Autodesk Inventor part; units mm, degrees
ref_plane "YZ Plane" through (0, 0, 0) normal (1, 0, 0) x (0, 1, 0)
ref_plane "XZ Plane" through (0, 0, 0) normal (0, 1, 0) x (-1, 0, 0)
ref_plane "XY Plane" through (0, 0, 0) normal (0, 0, 1) x (1, 0, 0)
sketch "Sketch1" plane through (0, 0, 0) normal (0, 0, 1) x (1, 0, 0)
  line L0 (33.401, 0) -> (-33.401, 0) construction
  arc A0 (33.401, 7.9375) -> (35.033, -7.7679) centre (33.401, 0) ccw construction
  arc A1 (-35.033, -7.7679) -> (-33.401, 7.9375) centre (-33.401, 0) ccw construction
  line L1 (33.401, 7.9375) -> (-33.401, 7.9375)
  line L2 (35.033, -7.7679) -> (19.1135, -11.1125)
  line L3 (19.1135, -11.1125) -> (19.1135, -30.1625)
  line L4 (19.1135, -30.1625) -> (44.5135, -36.9684)
  line L5 (44.5135, -36.9684) -> (44.5135, -81.4184)
  line L6 (44.5135, -81.4184) -> (-19.1135, -42.8625)
  line L7 (-19.1135, -42.8625) -> (-19.1135, -11.1125)
  line L8 (-19.1135, -11.1125) -> (-43.434, -6.0029)
  arc A2 (35.033, -7.7679) -> (33.401, 7.9375) centre (33.401, 0) ccw
  arc A3 (-33.401, 7.9375) -> (-35.033, -7.7679) centre (-33.401, 0) ccw
  line L9 (0, 26.6914) -> (0, -99.4367) construction
  line L10 (-33.401, 7.9375) -> (-43.434, 7.9375)
  line L11 (-43.434, 7.9375) -> (-43.434, -6.0029)
  point P0 (0, 0)
  point P1 (0, 0)
  point P2 (19.1135, -20.6375)
  dimension "d24" = 50.927
  dimension "d25" = 7.9375
  dimension "d26" = 19.05
  dimension "d27" = 19.05
  dimension "d28" = 105
  dimension "d30" = 6.35
  dimension "d31" = 44.45
  dimension "d72" = 28.575
  dimension "d110" = 31.75
  dimension "d127" = 10.033
extrude "Extrusion2" add sketch "Sketch1" along normal mid plane 9.525
sketch "Sketch2" plane through (0, 0, 4.7625) normal (0, 0, 1) x (1, 0, 0)
  arc A0 (35.033, -7.7679) -> (33.401, 7.9375) centre (33.401, 0) ccw construction
  line L0 (33.401, 0) -> (-33.401, 0) construction
  point P0 (0, 0)
  point P1 (0, 0)
hole "Hole1" at (33.401, 0, 4.7625) at (-33.401, 0, 4.7625) direction (0, 0, -1) diameter 3.9624 end through all
sketch "Sketch3" plane through (0, 0, -4.7625) normal (0, 0, -1) x (-1, 0, 0)
  line L0 (-62.103, 0) -> (61.0235, 0) construction
  line L1 (0, -99.2896) -> (0, 25.8087) construction
  line L2 (11.1125, -1.5875) -> (-11.1125, -1.5875) construction
  line L3 (0, -26.9875) -> (0, -1.5875) construction
  point P0 (0, 0)
  dimension "d43" = 22.225
  dimension "d44" = 25.4
  dimension "d45" = 1.5875
hole "Hole2" at (0, -26.9875, -4.7625) at (11.1125, -1.5875, -4.7625) at (-11.1125, -1.5875, -4.7625) direction (0, 0, 1) diameter 3.9624 end through all
sketch "Sketch4" plane through (0, 0, 4.7625) normal (0, 0, 1) x (1, 0, 0)
  line L0 (0, 0) -> (0, -12.7) construction
  circle A0 centre (0, -12.7) radius 9.525
  line L1 (25.4635, -56.9863) -> (25.4635, -41.6407)
  line L2 (23.9574, -39.6779) -> (-0.5536, -33.1102)
  line L3 (-3.1115, -35.073) -> (-3.1115, -42.1335)
  line L4 (-2.1326, -43.8713) -> (22.3784, -58.7242)
  line L5 (-19.1135, -42.8625) -> (44.5135, -81.4184) construction
  line L6 (44.5135, -36.9684) -> (19.1135, -30.1625) construction
  line L7 (44.5135, -81.4184) -> (44.5135, -36.9684) construction
  arc A1 (22.3784, -58.7242) -> (25.4635, -56.9863) centre (23.4315, -56.9863) ccw
  arc A2 (25.4635, -41.6407) -> (23.9574, -39.6779) centre (23.4315, -41.6407) ccw
  arc A3 (-0.5536, -33.1102) -> (-3.1115, -35.073) centre (-1.0795, -35.073) ccw
  arc A4 (-3.1115, -42.1335) -> (-2.1326, -43.8713) centre (-1.0795, -42.1335) ccw
  point P0 (-18.2864, -30.0929)
  point P1 (20.2266, -29.9445)
  point P2 (19.1135, -30.1625)
  dimension "d54" = 19.05
  dimension "d55" = 12.7
  dimension "d56" = 19.05
  dimension "d57" = 28.575
  dimension "d58" = 7.9375
  dimension "d59" = 7.9375
  dimension "d60" = 2.032
extrude "Extrusion3" cut sketch "Sketch4" against normal through all
sketch "Sketch6" plane through (19.1135, -30.1625, 4.7625) normal (1, 0, 0) x (0, 0, -1)
  line L0 (9.525, 19.05) -> (0, 19.05) construction
  line L1 (0, 0) -> (0, 19.05) construction
  line L2 (9.525, 0) -> (0, 0) construction
  line L3 (9.525, 19.05) -> (9.525, 0) construction
  line L4 (9.525, 0) -> (0, 19.05) construction
  point P0 (4.7625, 30.1625)
  point P1 (4.7625, 9.525)
hole "Hole3" at (19.1135, -20.6375, 0) direction (-1, 0, 0) diameter 3.9624 end through all
sketch "Sketch8" plane through (0, 0, -4.7625) normal (0, 0, -1) x (-1, 0, 0)
  line L0 (-38.1635, -41.7309) -> (-38.1635, -48.0809) construction
  line L1 (-38.1635, -48.0809) -> (-38.1635, -60.7809) construction
  line L2 (-38.1635, -60.7809) -> (-38.1635, -67.1309) construction
  line L3 (-44.5135, -36.9684) -> (-44.5135, -81.4184) construction
  point P0 (0, 0)
  point P1 (-44.5135, -59.1934)
  point P2 (-38.1635, -54.4309)
  dimension "d85" = 12.7
  dimension "d86" = 25.4
  dimension "d88" = 4.7625
  dimension "d89" = 6.35
hole "Hole5" at (38.1635, -67.1309, -4.7625) at (38.1635, -41.7309, -4.7625) direction (0, 0, 1) diameter 5.0038 end through all
hole "Hole6" at (38.1635, -48.0809, -4.7625) at (38.1635, -60.7809, -4.7625) direction (0, 0, 1) diameter 5.1054 end through all
fillet "Fillet4" radius 1.5875 3 edges at (19.1135, -30.1625, 0) (19.1135, -11.1125, 0) (-19.1135, -11.1125, 0)
fillet "Fillet5" radius 3.175 5 edges at (44.5135, -36.9684, 0) (44.5135, -81.4184, 0) (-19.1135, -42.8625, 0) (-43.434, -6.0029, 0) (-43.434, 7.9375, 0)
sketch "Sketch11" plane through (-43.434, -3.4256, -4.7625) normal (-1, 0, 0) x (0, 0, 1)
  point P0 (4.7625, 3.4256)
  point P1 (4.7625, 3.4256)
hole "Hole9" at (-43.434, 0, 0) direction (1, 0, 0) diameter 3.9624 depth 6.35 tip angle 118
equation "\"d58\" = d59"
equation "\"BendRadius\" = Thickness"
equation "\"BendReliefWidth\" = Thickness"
equation "\"BendReliefDepth\" = 0.5 * Thickness"
equation "\"CornerReliefSize\" = 4 * Thickness"
equation "\"MinimumRemnant\" = 2 * Thickness"
equation "\"TransitionRadius\" = BendRadius"
equation "\"JacobiRadiusSize\" = BendRadius"
equation "\"GapSize\" = Thickness"
properties part number "PLATE,SIDE,ELEVATOR,STAGE1" material "Aluminum 7075"
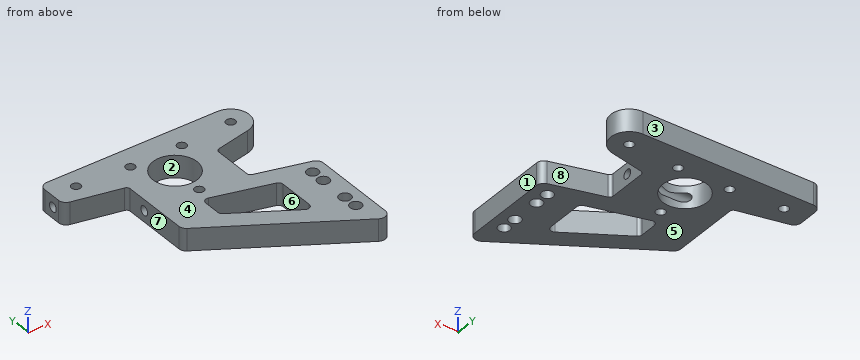
Design review of the part built by this model. Coordinates are the model's own, in mm. Face numbers are marked on the shaded views. A direction names the side the tool comes from. Coordinates: 2 decimals unless noted, no trailing zeros. Order: outer loops, then holes, each group sorted by start corner. A loop starts at its lowest first (then second) coordinate and runs counter-clockwise, first axis right, second up. Notation, with made-up numbers: (-18, -4.75) -> (-5, -4.75) arc R25 ccw to (-5, 29.25) -> close; hole circle Ø10 at (54.5, 67.25). An arc over 180 degrees is marked (long way). One line per item, written item: value. Start each with the question number.
Q1. For probe 1 along Z at (x, y) = (-39.5, 0); probe 2 along X at (y, z) = (-49.5, -4); probe 3 along Y at (x, z) = (21.5, -2.25), list the stretches that pass through material, from the lowest coordinate up.
Q2. Insertion check: pin 1 Ø5 at (y, z) = (-35, -0.5) entering from +X; pin 2 Ø3 at (y, z) = (-59.5, -2) entering from -X; pin 3 Ø2.5 at (y, z) = (0, 0) entering from +X. Each pin has a flat end and moves straight along its axis. Give the tip position at first contact, or say it passes through.
Q3. Take a section at A-A, the plane x = -26.5. State the section outline as (y, z) points.
Q4. Take a section at B-B, the plane y = -72. State the section outline as (x, z) points, then the cut area to 3 significant figures.
Q5. Tool access review of the marked faces 4, 5, 6, 7 and 8: name each direction out of +Z, -Z, +X, -X, +Y, -Y from which nothing blocks a thin tool from reaching the whole face with its end or side.
Q6. Mouldability with a two-part tool opening along X and no side actions: class the marked faces 1, 2 and 3 as pulls with the +X half, pulls with the -X half, needs draft (parallel to the pull), parting line crosses it, or undercut.
Values follow:
1. probe 1: z = -4.76 to -1.98, 1.98 to 4.76
1. probe 2: x = -8.16 to 7.16, 25.46 to 36.04, 40.29 to 44.51
1. probe 3: y = -67.47 to -58.19, -39.02 to -30.8, -10.61 to 7.94
2. pin 1: stops at x = 43.88
2. pin 2: stops at x = 5.87
2. pin 3: stops at x = 41.34
3. outline: (-9.56, -4.76) -> (7.94, -4.76) -> (7.94, 4.76) -> (-9.56, 4.76) -> close
4. outline: (28.97, -4.76) -> (44.51, -4.76) -> (44.51, 4.76) -> (28.97, 4.76) -> close
4. area: 148 mm2
5. face 4: +Z, +X, -X, +Y, -Y
5. face 5: -Z, +X, -X, +Y, -Y
5. face 6: +Z, -Z
5. face 7: +Z, -Z, -X, -Y
5. face 8: +Z, -Z, +X
6. face 1: pulls with the +X half
6. face 2: undercut
6. face 3: needs draft
